Input: part model. Units: mm. Frame: model coordinates. Face numbers are marked on the shaded views. A direction names the side the tool comes from. Round coordinates to 2 decimals unless told otherwise and drop trailing zeros. Order: outer loops, then holes, each group sorted by start corner. A loop starts at its lowest first (then second) coordinate and runs counter-clockwise, first axis right, second up.
Item 1: Reachability of the marked faces 1 and 2 from +Z, -Z, +X, -X, +Y, -Y: full face, straight path, thin tool, end or side. Return the list, or none.
Item 2: First-contact query: pin 1 (3 mm diameter, centred on y = -4.5, z = 11, fed in from +X); pin 2 (6 mm diameter, centred on y = 3.5, z = 3.5, fed in from +X); pin 3 (3 mm diameter, centred on y = 5, z = 3, fed in from -X). Flat tips, straight axial feed; report the tip coordinate or a pass-through.
Item 3: Cut plane D-D on z = 8. Output: boundary loops of the cut face in (x, y), then the cut area to 3 significant figures.
Item 4: Cut plane A-A on x = 0. Output: boundary loops of the cut face in (y, z) (3 decimals).
Item 5: Line query: L1, parallel to Z at x = -0.5, y = 6.75; L2, parallel to X at y = -0.75, z = 14; L3, parallel to X at y = 1.5, z = 11. Output: solid intervals per line, ascending.
Item 6: Cut plane C-C on x = -6. Output: boundary loops of the cut face in (y, z), then the cut area to 3 significant figures.
```python
from build123d import *

# Parameters (mm, degrees)
SKETCH1_R                = 5.22
BOSS_EXTRUDE1_DEPTH      = 28
SKETCH2_R                = 7
BOSS_EXTRUDE2_DEPTH      = 4
CUT_EXTRUDE2_START       = -3
CUT_EXTRUDE2_OUTLINE_R   = 7
CUT_EXTRUDE2_OUTLINE_R_2 = 5.165
CUT_EXTRUDE2_DEPTH       = 1


# Read off the part's stored shape, not the designer's step: Cut-Extrude2
with BuildPart() as part:
    # Sketch1 → Boss-Extrude1 (new body)
    with BuildSketch(Plane.XY):
        Circle(SKETCH1_R)
    extrude(amount=BOSS_EXTRUDE1_DEPTH)

    # Sketch2 → Boss-Extrude2 (add)
    with BuildSketch(Plane(origin=(0, 0, 0), x_dir=(-1, 0, 0), z_dir=(0, 0, -1))):
        Circle(SKETCH2_R)
    extrude(amount=BOSS_EXTRUDE2_DEPTH)

    # Cut-Extrude2 outline → Cut-Extrude2 (cut)
    with BuildSketch(Plane.XY.offset(CUT_EXTRUDE2_START)):
        Circle(CUT_EXTRUDE2_OUTLINE_R)
        Circle(CUT_EXTRUDE2_OUTLINE_R_2, mode=Mode.SUBTRACT)
    extrude(amount=CUT_EXTRUDE2_DEPTH, mode=Mode.SUBTRACT)


solid = part.part
```
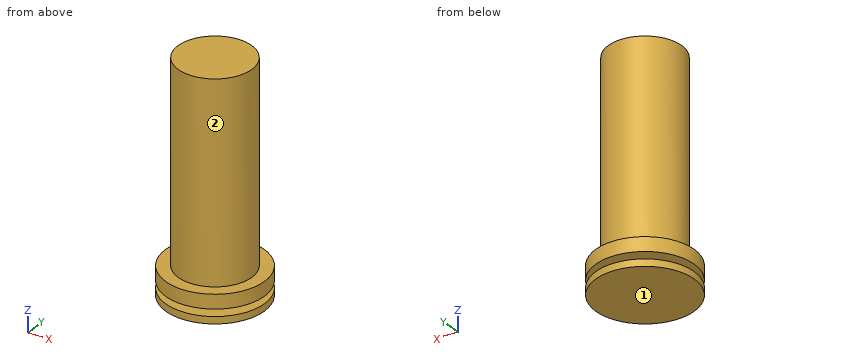
From the geometry:
1. face 1: -Z, +X, -X, +Y, -Y
1. face 2: +Z
2. pin 1: stops at x = 4.27
2. pin 2: stops at x = 5.2
2. pin 3: stops at x = -3.87
3. outline: circle Ø10.44 at (0, 0)
3. area: 85.6 mm2
4. outline: (-7, -4) - (7, -4) - (7, -3) - (5.165, -3) - (5.165, -2) - (7, -2) - (7, 0) - (5.22, 0) - (5.22, 28) - (-5.22, 28) - (-5.22, 0) - (-7, 0) - (-7, -2) - (-5.165, -2) - (-5.165, -3) - (-7, -3) - close
5. L1: z = -4 to -3, -2 to 0
5. L2: x = -5.17 to 5.17
5. L3: x = -5 to 5
6. outline: (-3.61, -4) - (3.61, -4) - (3.61, -3) - (-3.61, -3) - close; (-3.61, -2) - (3.61, -2) - (3.61, 0) - (-3.61, 0) - close
6. area: 21.6 mm2
